For this review, take the finished solid that the model builds, in its own axes (mm). Give positions to 0.01 mm unless a question says otherwise; leave off trailing zeros. Order: outer loops, then holes, each group sorted by start corner. A loop starts at its lowest first (then second) coordinate and runs counter-clockwise, first axis right, second up. Notation, with made-up numbers: (7.25, -13.5) - (13.25, -13.5) arc R17 cw to (13.25, 4.5) - close; hole circle Ø10 at (7.5, 69.25). An arc over 180 degrees is marked (long way). Put each result on its own line as item: value. Start each with the question number.
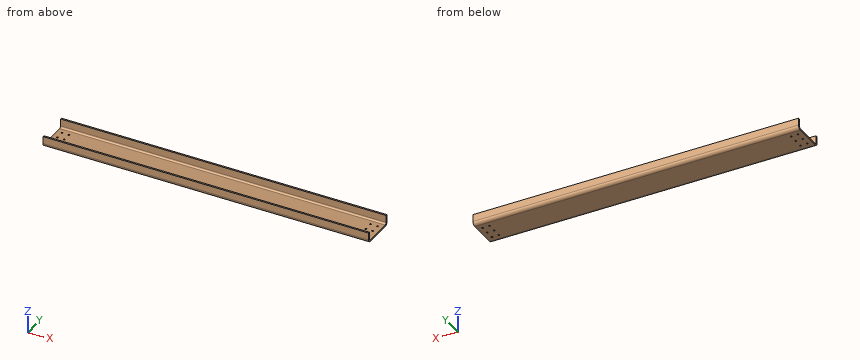
Autodesk Inventor part; units mm, degrees
ref_plane "YZ Plane" through (0, 0, 0) normal (1, 0, 0) x (0, 1, 0)
ref_plane "XZ Plane" through (0, 0, 0) normal (0, 1, 0) x (-1, 0, 0)
ref_plane "XY Plane" through (0, 0, 0) normal (0, 0, 1) x (1, 0, 0)
sketch "Sketch2" plane through (0, 0, 0) normal (0, 0, 1) x (1, 0, 0)
  line L0 (-301.752, 25.273) -> (301.752, 25.273)
  line L1 (301.752, 25.273) -> (301.752, -25.273)
  line L2 (301.752, -25.273) -> (-301.752, -25.273)
  line L3 (-301.752, -25.273) -> (-301.752, 25.273)
  point P0 (0, 0)
  dimension "d0" = 301.752
  dimension "d1" = 301.752
  dimension "d2" = 25.273
  dimension "d3" = 25.273
extrude "Plate1" add sketch "Sketch2" along normal blind 3.048
sketch "Sketch3" plane through (301.752, -25.273, 0) normal (1, 0, 0) x (0, 0, -1)
  line L0 (0, 50.546) -> (-3.048, 50.546)
  arc A0 (0, 50.546) -> (-6.223, 56.769) centre (-6.223, 50.546) ccw
  line L1 (-6.223, 50.546) -> (-6.223, 56.769) construction
  line L2 (-6.223, 50.546) -> (0, 50.546) construction
  line L3 (-6.223, 56.769) -> (-19.5834, 56.769)
  point P0 (0, 25.273)
  dimension "d5" = 90
  dimension "d6" = 6.223
  dimension "d7" = 6.223
  dimension "d8" = 13.3604
contour flange "Contour Flange1" sketch "Sketch3" thickness 3.048 bend radius 3.048 curves A0 L3 edges at (0, 25.273, 0) running between points at (-301.752, 25.273, 0) (301.752, 25.273, 0)
bend "Bend1"
corner "Corner1"
sketch "Sketch4" plane through (301.752, -25.273, 3.048) normal (1, 0, 0) x (0, 0, -1)
  line L0 (3.048, 0) -> (0, 0)
  arc A0 (-3.175, -6.223) -> (3.048, 0) centre (-3.175, 0) ccw
  line L1 (-3.175, 0) -> (-3.175, -6.223) construction
  line L2 (-3.175, 0) -> (3.048, 0) construction
  line L3 (-3.175, -6.223) -> (-16.5354, -6.223)
  point P0 (3.048, 25.273)
  dimension "d18" = 90
  dimension "d19" = 6.223
  dimension "d20" = 6.223
  dimension "d21" = 13.3604
contour flange "Contour Flange2" sketch "Sketch4" thickness 3.048 bend radius 3.048 curves L3 A0 edges at (0, -25.273, 0) running between points at (301.752, -25.273, 0) (-301.752, -25.273, 0)
bend "Bend2"
corner "Corner2"
sketch "Sketch5" plane through (0, 0, 0) normal (0, 0, -1) x (-1, 0, 0)
  line L0 (-301.752, 25.273) -> (-301.752, -25.273)
  line L1 (-301.752, -25.273) -> (301.752, -25.273)
  line L2 (301.752, -25.273) -> (301.752, 25.273)
  point P0 (0, 0)
  point P1 (-292.354, -15.748)
  point P2 (279.654, -15.748)
  dimension "d31" = 9.398
  dimension "d32" = 22.098
  dimension "d33" = 9.525
  dimension "d34" = 9.525
hole "Hole1" at (292.354, -15.748, 0) at (-279.654, -15.748, 0) direction (0, 0, 1) diameter 3.175 end through all
sketch "Sketch6" plane through (0, 0, 0) normal (0, 0, -1) x (-1, 0, 0)
  circle A0 centre (-292.354, -15.748) radius 1.5875
  line L0 (301.752, -25.273) -> (301.752, 25.273)
  line L1 (-292.354, -15.748) -> (-277.2602, -15.748)
  point P0 (0, 0)
sketch "Sketch7" plane through (0, 0, 0) normal (0, 0, -1) x (-1, 0, 0)
  circle A0 centre (-292.354, -15.748) radius 1.5875
  line L0 (301.752, -25.273) -> (301.752, 25.273)
  line L1 (-292.354, -15.748) -> (-292.354, -4.4863)
  point P0 (0, 0)
pattern_linear "Rectangular Pattern1" count 2 spacing 12.7 along (-1, 0, 0) count 3 spacing 15.748 along (0, 1, 0) of "Hole1"
equation "\"d40\" = Thickness"
equation "\"d9\" = BendReliefWidth"
equation "\"d10\" = BendReliefDepth"
equation "\"d11\" = MinimumRemnant"
equation "\"d12\" = BendRadius"
equation "\"d13\" = BendRadius"
equation "\"d15\" = CornerReliefSize"
equation "\"d16\" = GapSize"
equation "\"d17\" = JacobiRadiusSize"
equation "\"d22\" = BendReliefWidth"
equation "\"d23\" = BendReliefDepth"
equation "\"d24\" = MinimumRemnant"
equation "\"d25\" = BendRadius"
equation "\"d26\" = BendRadius"
equation "\"d28\" = CornerReliefSize"
equation "\"d29\" = GapSize"
equation "\"d30\" = JacobiRadiusSize"
equation "\"BendRadius\" = Thickness"
equation "\"BendReliefWidth\" = Thickness"
equation "\"BendReliefDepth\" = 0.5 * Thickness"
equation "\"CornerReliefSize\" = 4 * Thickness"
equation "\"MinimumRemnant\" = 2 * Thickness"
equation "\"TransitionRadius\" = BendRadius"
equation "\"JacobiRadiusSize\" = BendRadius"
equation "\"GapSize\" = Thickness"
equation "\"d4\" = BendRadius"
properties part number "Base Back Bar"
1. Add section B-B, the plane x = -240. Give the boundary of the cut face in (y, z) (3 decimals).
2. Add section C-C, the plane y = -7.5. Give the boundary of the cut face in (x, z).
3. Add section A-A, the plane z = 13.75. Give the boundary of the cut face in (x, y).
4. Wall thickness on line 1 (X direction, y = 0, z = 1.8); line 2 (Y direction, x = -218.5, z = 15); line 3 (Z direction, x = 73, y = -6.5): over which ranges is each line inside the solid? List them lowest first. Write a range as from..to.
5. Clearance check with a flat-ended pin moving along its axis: pin 1 (5 mm diameter, centred on x = 292.354, y = 15.748, fed in from +Z). State where the tip first meets the part, or that it passes through.
Found:
1. outline: (-31.496, 6.223) arc R6.223 ccw to (-25.273, 0) - (25.273, 0) arc R6.223 ccw to (31.496, 6.223) - (31.496, 19.583) - (28.448, 19.583) - (28.448, 6.223) arc R3.175 cw to (25.273, 3.048) - (-25.273, 3.048) arc R3.175 cw to (-28.448, 6.223) - (-28.448, 19.583) - (-31.496, 19.583) - close
2. outline: (-301.75, 0) - (301.75, 0) - (301.75, 3.05) - (-301.75, 3.05) - close
3. outline: (-301.75, -31.5) - (301.75, -31.5) - (301.75, -28.45) - (-301.75, -28.45) - close; (-301.75, 28.45) - (301.75, 28.45) - (301.75, 31.5) - (-301.75, 31.5) - close
4. line 1: x = -301.75..-293.94, -290.77..-281.24, -278.07..278.07, 281.24..290.77, 293.94..301.75
4. line 2: y = -31.5..-28.45, 28.45..31.5
4. line 3: z = 0..3.05
5. pin 1: stops at z = 3.05
